from build123d import *

# Parameters (mm, degrees)
IZIM1_W                     = 23.2
IZIM1_H                     = 7.3
Y_KSEKLIK_EKSTR_ZYON1_DEPTH = 401.7
KES_EKSTR_ZYON1_DEPTH       = 402.7
KES_EKSTR_ZYON2_DEPTH       = 402.7
KES_EKSTR_ZYON3_DEPTH       = 402.7


with BuildPart() as part:
    # Çizim1 → Yükseklik-Ekstrüzyon1 (new body)
    with BuildSketch(Plane.XY):
        with Locations((11.6, 3.65)):
            Rectangle(IZIM1_W, IZIM1_H)
    extrude(amount=Y_KSEKLIK_EKSTR_ZYON1_DEPTH)

    # Çizim2 → Kes-Ekstrüzyon1 (cut)
    with BuildSketch(Plane.XY.offset(401.7)):
        Polygon((21.2, 7.3), (23.2, 7.3), (23.2, 4.3), (21.2, 4.3), (21.2, 6.3), (0, 6.3), (0, 7.3), align=None)
        Polygon((0, 0), (2, 0), (23.2, 0), (23.2, 1), (2, 1), (2, 3), (0, 3), align=None)
    extrude(amount=-KES_EKSTR_ZYON1_DEPTH, mode=Mode.SUBTRACT)

    # Çizim3 → Kes-Ekstrüzyon2 (cut)
    with BuildSketch(Plane(origin=(0, 6.3, 0), x_dir=(1, 0, 0), z_dir=(0, 1, 0))):
        with BuildLine():
            Line((0, 0), (5.6, 0))
            add(Edge.make_bspline(
                [(5.6, 0), (0.42062512, -27.8813272), (0, -56)],
                knots=[0, 0, 0, 0.849776743, 0.849776743, 0.849776743], degree=2))
            Line((0, -56), (0, 0))
        make_face()
        with BuildLine():
            Line((23.2, 0), (23.2, -56))
            add(Edge.make_bspline(
                [(17.6, 0), (22.77937488, -27.8813272), (23.2, -56)],
                knots=[0, 0, 0, 0.849776743, 0.849776743, 0.849776743], degree=2))
            Line((17.6, 0), (23.2, 0))
        make_face()
    extrude(amount=-KES_EKSTR_ZYON2_DEPTH, mode=Mode.SUBTRACT)

    # Çizim4 → Kes-Ekstrüzyon3 (cut)
    with BuildSketch(Plane(origin=(0, 6.3, 0), x_dir=(1, 0, 0), z_dir=(0, 1, 0))):
        with BuildLine():
            Line((8.2, -27.6), (8.2, -76.8))
            ThreePointArc((8.2, -76.8), (11.6, -80.2), (15, -76.8))
            Line((15, -76.8), (15, -27.6))
            ThreePointArc((15, -27.6), (11.6, -24.2), (8.2, -27.6))
        make_face()
        with BuildLine():
            Line((8.2, -99.4), (8.2, -148.6))
            ThreePointArc((8.2, -148.6), (11.6, -152), (15, -148.6))
            Line((15, -148.6), (15, -99.4))
            ThreePointArc((15, -99.4), (11.6, -96), (8.2, -99.4))
        make_face()
        with BuildLine():
            Line((8.2, -211.4), (8.2, -260.6))
            ThreePointArc((8.2, -260.6), (11.6, -264), (15, -260.6))
            Line((15, -260.6), (15, -211.4))
            ThreePointArc((15, -211.4), (11.6, -208), (8.2, -211.4))
        make_face()
        with BuildLine():
            Line((8.2, -283.2), (8.2, -332.4))
            ThreePointArc((8.2, -332.4), (11.6, -335.8), (15, -332.4))
            Line((15, -332.4), (15, -283.2))
            ThreePointArc((15, -283.2), (11.6, -279.8), (8.2, -283.2))
        make_face()
    extrude(amount=-KES_EKSTR_ZYON3_DEPTH, mode=Mode.SUBTRACT)


solid = part.part
The model under review builds one solid part; all positions refer to its coordinate system, in mm. Round coordinates to 2 decimals unless told otherwise and drop trailing zeros. Loops run counter-clockwise (first coordinate to the right, second up) from the corner with the lowest first, then second, coordinate; pieces in that order, holes last. Notation, with made-up numbers: (0.25, 34) -> (34.25, 34) arc R26 cw to (34.25, 52) -> close; hole circle Ø11 at (31, 29.5). An arc over 180 degrees is marked (long way). Return JSON: item names as keys, results as strings.
(1) For pin 1 (2 mm diameter, centred on y = 1.5, z = 170, fed in from -X); pin 2 (2 mm diameter, centred on x = 0.5, z = 149.5, fed in from -Y); pin 3 (1 mm diameter, centred on y = 5.5, z = 342.5, fed in from +X), all flat-tipped, find the tip position at first contact; note any pin that passes through.
Solved:
{"pin 1": "x = 2", "pin 2": "y = 3", "pin 3": "x = 21.2"}
(2) Add section B-B on x = 11.6. Write out the cut boundary in (y, z).
Solved:
{"outline": "(1, 0) -> (6.3, 0) -> (6.3, 24.2) -> (1, 24.2) -> close; (1, 80.2) -> (6.3, 80.2) -> (6.3, 96) -> (1, 96) -> close; (1, 152) -> (6.3, 152) -> (6.3, 208) -> (1, 208) -> close; (1, 264) -> (6.3, 264) -> (6.3, 279.8) -> (1, 279.8) -> close; (1, 335.8) -> (6.3, 335.8) -> (6.3, 401.7) -> (1, 401.7) -> close"}
(3) Add section C-C on z = 174.5. Write out the cut boundary in (x, y).
Solved:
{"outline": "(0, 3) -> (2, 3) -> (2, 1) -> (23.2, 1) -> (23.2, 4.3) -> (21.2, 4.3) -> (21.2, 6.3) -> (0, 6.3) -> close"}
(4) Add section D-D on y = 5.45. State how many separate pieces and enclosed holes the cut face has, plus the area to 3 significant figures.
Solved:
{"separate pieces": "1", "enclosed holes": "4", "area": "6,880 mm2"}
(5) For line 1 (Z direction, x = 11.5, y = 3.3); line 2 (Z direction, x = 11, y = 2.15); line 3 (X direction, y = 2.2, z = 71), list the stretches that pass through material, from the lowest coordinate up.
Solved:
{"line 1": "0 to 24.2, 80.2 to 96, 152 to 208, 264 to 279.8, 335.8 to 401.7", "line 2": "0 to 24.25, 80.15 to 96.05, 151.95 to 208.05, 263.95 to 279.85, 335.75 to 401.7", "line 3": "2 to 8.2, 15 to 23.2"}
(6) Add section A-A on z = 301. Write out the cut boundary in (x, y).
Solved:
{"outline": "(0, 3) -> (2, 3) -> (2, 1) -> (8.2, 1) -> (8.2, 6.3) -> (0, 6.3) -> close; (15, 1) -> (23.2, 1) -> (23.2, 4.3) -> (21.2, 4.3) -> (21.2, 6.3) -> (15, 6.3) -> close"}
